from build123d import *

# Parameters (mm, degrees)
F0_W      = 269.38311
F0_H      = 16.098589
F0_H_2    = 69.402822
F1_DEPTH  = 68.58
F2_W      = 269.38311
F2_H      = 13.501506
F3_DEPTH  = 51.816
F4_W      = 55.430394
F4_H      = 9.777048
F5_DEPTH  = 176.784
F6_DEPTH  = 15.24
F7_W      = 55.430394
F7_H      = 9.777048
F8_DEPTH  = 26.416
F9_W      = 39.127992
F9_H      = 11.603475
F10_DEPTH = 187.198


with BuildPart() as f1:
    # F0 (on Top) → F1 (new body)
    with BuildSketch(Plane.XY):
        with Locations((0, 42.750705)):
            Rectangle(F0_W, F0_H)
        Rectangle(F0_W, F0_H_2)
        with Locations((0, -42.750705)):
            Rectangle(F0_W, F0_H)
    extrude(amount=F1_DEPTH)

    # F2 (on face) → F3 (cut)
    with BuildSketch(Plane.XY.offset(68.58)):
        Rectangle(F2_W, F2_H)
    extrude(amount=-F3_DEPTH, mode=Mode.SUBTRACT)

    # F4 (on face) → F5 (cut)
    with BuildSketch(Plane.YZ.offset(134.691555)):
        with Locations((-0.261033, 15.165092)):
            Rectangle(F4_W, F4_H)
    extrude(amount=-F5_DEPTH, mode=Mode.SUBTRACT)

    # F4 (on face) → F6 (join)
    with BuildSketch(Plane.YZ.offset(134.691555)):
        with Locations((-0.261033, 15.165092)):
            Rectangle(F4_W, F4_H)
    extrude(amount=-F6_DEPTH)

    # F7 (on face) → F8 (join)
    with BuildSketch(Plane(origin=(-134.691555, 0, 0), x_dir=(0, -1, 0), z_dir=(-1, 0, 0))):
        with Locations((20.964444, 15.165092)):
            Rectangle(F7_W, F7_H)
    extrude(amount=-F8_DEPTH)

    # F9 (on face) → F10 (cut)
    with BuildSketch(Plane.YZ.offset(134.691555)):
        with Locations((0.539697, 17.944907)):
            Rectangle(F9_W, F9_H)
    extrude(amount=-F10_DEPTH, mode=Mode.SUBTRACT)


solid = f1.part
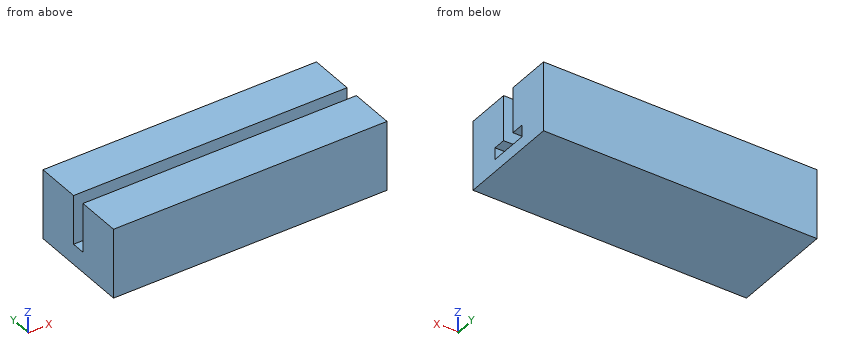
For this review, take the finished solid that the model builds, in its own axes (mm). Coordinates: 2 decimals unless noted, no trailing zeros. Loops run counter-clockwise (first coordinate to the right, second up) from the corner with the lowest first, then second, coordinate; pieces in that order, holes last. Notation, with made-up numbers: (-9, 11.25) - (2, 11.25) arc R29 cw to (2, 41.25) - close; hole circle Ø2 at (53, -2). An arc over 180 degrees is marked (long way). Return JSON: item names as keys, results as strings.
Item 1: Take a section at B-B (x = 98.5). Give the boundary of the cut face in (y, z), then the cut area to 3 significant figures.
Determined:
{"outline": "(-50.8, 0) - (50.8, 0) - (50.8, 68.58) - (6.75, 68.58) - (6.75, 23.75) - (20.1, 23.75) - (20.1, 20.05) - (27.45, 20.05) - (27.45, 10.28) - (-27.98, 10.28) - (-27.98, 20.05) - (-19.02, 20.05) - (-19.02, 23.75) - (-6.75, 23.75) - (-6.75, 68.58) - (-50.8, 68.58) - close", "area": "5,680 mm2"}
Item 2: For line 1 (Y direction, x = 115.5, z = 14.5); line 2 (Y direction, x = 60.5, z = 58); line 3 (Z direction, x = -40.5, y = -21.5), list the stretches that pass through material, from the lowest coordinate up.
Determined:
{"line 1": "y = -50.8 to -27.98, 27.45 to 50.8", "line 2": "y = -50.8 to -6.75, 6.75 to 50.8", "line 3": "z = 0 to 10.28, 20.05 to 68.58"}
Item 3: Take a section at A-A (z = 35). Give the boundary of the cut face in (x, y).
Determined:
{"outline": "(-134.69, -50.8) - (134.69, -50.8) - (134.69, -6.75) - (-134.69, -6.75) - close; (-134.69, 6.75) - (134.69, 6.75) - (134.69, 50.8) - (-134.69, 50.8) - close"}
Item 4: Take a section at C-C (y = -14.5). Give the boundary of the cut face in (x, z).
Determined:
{"outline": "(-134.69, 0) - (134.69, 0) - (134.69, 12.14) - (119.45, 12.14) - (119.45, 10.28) - (-42.09, 10.28) - (-42.09, 12.14) - (-52.51, 12.14) - (-52.51, 23.75) - (134.69, 23.75) - (134.69, 68.58) - (-134.69, 68.58) - close"}
Item 5: Insertion check: pin 1 (3 mm diameter, centred on x = -48, y = -2, fed in from +Z); pin 2 (6 mm diameter, centred on y = 4, z = 20, fed in from +X); pin 3 (2.5 mm diameter, centred on y = 1, z = 19, fed in from +X). Each pin has a flat end and moves straight along its axis. Give the tip position at first contact, or say it passes through.
Determined:
{"pin 1": "stops at z = 12.14", "pin 2": "stops at x = -52.51", "pin 3": "stops at x = -108.28"}
Item 6: Take a section at D-D (x = -113). Give the boundary of the cut face in (y, z), then the cut area to 3 significant figures.
Determined:
{"outline": "(-50.8, 0) - (50.8, 0) - (50.8, 68.58) - (6.75, 68.58) - (6.75, 20.05) - (-6.75, 20.05) - (-6.75, 68.58) - (-50.8, 68.58) - close", "area": "6,310 mm2"}
